Autodesk Inventor part; units mm, degrees
ref_plane "YZ Plane" through (0, 0, 0) normal (1, 0, 0) x (0, 1, 0)
ref_plane "XZ Plane" through (0, 0, 0) normal (0, 1, 0) x (-1, 0, 0)
ref_plane "XY Plane" through (0, 0, 0) normal (0, 0, 1) x (1, 0, 0)
sketch "Sketch1" plane through (0, 0, 0) normal (0, 1, 0) x (-1, 0, 0)
  line L0 (0, 0) -> (-19.05, 0)
  line L1 (-19.05, 0) -> (-19.05, 50.8)
  line L2 (-19.05, 50.8) -> (0, 50.8)
  line L3 (0, 50.8) -> (0, 0)
  circle A0 centre (-9.525, 3.175) radius 6.35
  point P0 (-1.5875, 0)
  point P1 (-11.1125, 0)
  dimension "d1" = 19.05
  dimension "d4" = 50.8
  dimension "d11" = 12.7
  dimension "d12" = 3.175
  dimension "d13" = 9.525
extrude "Extrusion1" add sketch "Sketch1" along normal blind 3.175 contours L0 A0 L1 L2 L3 | L0 A0 picked at (-8.7548, 5.6041)
sketch "Sketch2" plane through (0, 3.175, 0) normal (0, 1, 0) x (1, 0, 0)
  line L0 (17.4625, -49.2125) -> (17.4625, -39.6875) construction
  line L1 (19.05, -49.2125) -> (19.05, -39.6875)
  line L2 (15.875, -39.6875) -> (15.875, -49.2125)
  arc A0 (15.875, -49.2125) -> (19.05, -49.2125) centre (17.4625, -49.2125) ccw
  arc A1 (19.05, -39.6875) -> (15.875, -39.6875) centre (17.4625, -39.6875) ccw
  line L3 (0, -50.8) -> (19.05, -50.8)
  line L4 (19.05, -50.8) -> (19.05, 0)
  point P0 (0, 0)
  point P1 (17.4625, -44.45)
  dimension "d23" = 1.5875
  dimension "d24" = 1.5875
  dimension "d25" = 9.525
  dimension "d26" = 0
extrude "Extrusion2" add sketch "Sketch2" along normal blind 12.7 contours A0 L2 A1 L1
hole "Hole1" at (9.9145, 3.175, 1.4669) direction (0, -1, 0) diameter 10.4588 end through all
properties part number "piston locking tool"
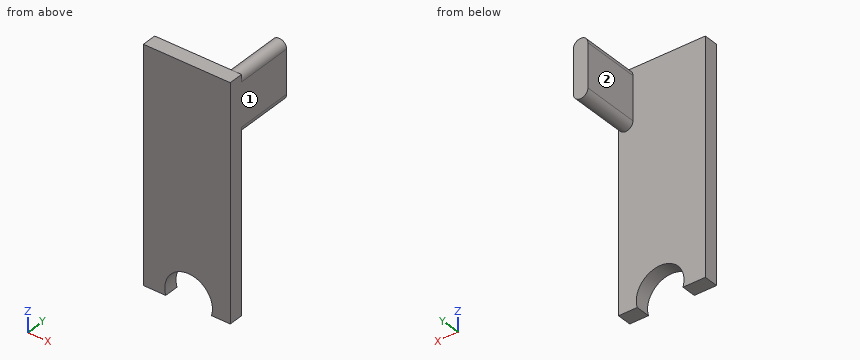
Verification items for the finished model (mm, model axes). Face numbers are marked on the shaded views. A direction names the side the tool comes from. Give positions to 0.01 mm unless a question says otherwise; leave off trailing zeros. Write each loop counter-clockwise with the first axis right and the second up, starting at its lowest first coordinate (ties: lowest second). Pieces come first, ordered by that corner, then holes. Notation, with made-up numbers: M 11,31 L 67,31 A18 cw 67,49 Z; hole C 71,65.5 d2. An arc over 180 degrees is marked long. Put each result on its own line as item: value. Start each with the question number.
1. Go/stop test with flat-tipped pins: pin 1 Ø4 at (y, z) = (6.5, 29) entering from +X; pin 2 Ø1.7 at (x, z) = (18.5, 50.5) entering from +Y (3 decimals); pin 3 Ø5 at (y, z) = (6.5, 45) entering from -X (3 decimals); pin 4 Ø5 at (x, z) = (12.5, 6) entering from +Y (3 decimals). Record where each tip stops, or that it passes through.
2. Section check C-C (z = 10). Record the cut outline in (x, y) (3 decimals).
3. Set-up check for the marked faces 1 and 2: record each of +Z, -Z, +X, -X, +Y, -Y from which the full face is reachable in a straight line by a thin tool's end or side.
4. Section check B-B (y = 2.5). Record the cut outline in (x, z).
5. Scan lines: line 1 along Y through (x, z) = (14, 10) (3 decimals); line 2 along X through (y, z) = (9.75, 41) (3 decimals); line 3 along Z through (x, y) = (11, 2.75). Record each from-to range of solid material in increasing order. Write a range as [from, to].
6. Section check D-D (x = 12.5). Record the cut outline in (y, z) (3 decimals), and give its area (3 significant figures).
7. Section check A-A (z = 4). Record the cut outline in (x, y) (3 decimals), and give its area (3 significant figures).
Answer list:
1. pin 1: through
1. pin 2: y = 15.875
1. pin 3: x = 15.875
1. pin 4: y = 3.175
2. outline: M 0,0 L 19.05,0 L 19.05,3.175 L 0,3.175 Z
3. face 1: +Z, -Z, +X, +Y, -Y
3. face 2: +Z, -Z, -X, +Y
4. outline: M 0,0 L 4.9,0 A5.23 cw long 14.93,0 L 19.05,0 L 19.05,50.8 L 0,50.8 Z
5. line 1: [0, 3.175]
5. line 2: [15.875, 19.05]
5. line 3: [6.58, 50.8]
6. outline: M 0,6.012 L 3.175,6.012 L 3.175,50.8 L 0,50.8 Z
6. area: 142 mm2
7. outline: M 0,0 L 5.34,0 L 5.34,3.175 L 0,3.175 Z; M 14.489,0 L 19.05,0 L 19.05,3.175 L 14.489,3.175 Z
7. area: 31.4 mm2
